For this review, take the finished solid that the model builds, in its own axes (mm). A direction names the side the tool comes from. Coordinates: 2 decimals unless noted, no trailing zeros. Order: outer loops, then holes, each group sorted by start corner. A loop starts at its lowest first (then second) coordinate and runs counter-clockwise, first axis right, second up. Notation, with made-up numbers: M 23.25,-12.75 L 50.25,-12.75 A32 ccw 50.25,17.25 Z; hole C -30,-10 d4. An arc over 180 degrees is marked long. Use CSV: the item, a comma, the result in double quotes.
```python
from build123d import *

# Parameters (mm, degrees)
ESBO_O1_R                = 5
RESSALTO_EXTRUS_O1_DEPTH = 8
ESBO_O1_3_R              = 2.5
RESSALTO_EXTRUS_O2_DEPTH = 4


with BuildPart() as part:
    # Esbo_o1 → Ressalto-extrus_o1 (new body)
    # profile 1 of 8: a face of its own
    with BuildSketch(Plane(origin=(0, 0, 0), x_dir=(1, 0, 0), z_dir=(0, 1, 0))):
        Polygon((8.06917925, -4.658742812), (8.06917925, 4.658742812), (0, 9.317485624), (-8.06917925, 4.658742812), (-8.06917925, -4.658742812), (0, -9.317485624), align=None)
        Circle(ESBO_O1_R, mode=Mode.SUBTRACT)
    # profile 2 of 8: a face of its own
    with BuildSketch(Plane(origin=(0, 0, 0), x_dir=(1, 0, 0), z_dir=(0, 1, 0))):
        Polygon((0, 9.317485624), (-4.658742812, 8.06917925), (-8.06917925, 4.658742812), align=None)
    # profile 3 of 8: a face of its own
    with BuildSketch(Plane(origin=(0, 0, 0), x_dir=(1, 0, 0), z_dir=(0, 1, 0))):
        Polygon((8.06917925, 4.658742812), (4.658742812, 8.06917925), (0, 9.317485624), align=None)
    # profile 4 of 8: a face of its own
    with BuildSketch(Plane(origin=(0, 0, 0), x_dir=(1, 0, 0), z_dir=(0, 1, 0))):
        Polygon((8.06917925, -4.658742812), (9.317485624, 0), (8.06917925, 4.658742812), align=None)
    # profile 5 of 8: a face of its own
    with BuildSketch(Plane(origin=(0, 0, 0), x_dir=(1, 0, 0), z_dir=(0, 1, 0))):
        Polygon((0, -9.317485624), (4.658742812, -8.06917925), (8.06917925, -4.658742812), align=None)
    # profile 6 of 8: a face of its own
    with BuildSketch(Plane(origin=(0, 0, 0), x_dir=(1, 0, 0), z_dir=(0, 1, 0))):
        Polygon((-8.06917925, -4.658742812), (-4.658742812, -8.06917925), (0, -9.317485624), align=None)
    # profile 7 of 8: a face of its own
    with BuildSketch(Plane(origin=(0, 0, 0), x_dir=(1, 0, 0), z_dir=(0, 1, 0))):
        Polygon((-8.06917925, 4.658742812), (-9.317485624, 0), (-8.06917925, -4.658742812), align=None)
    # profile 8 of 8: a face of its own
    with BuildSketch(Plane(origin=(0, 0, 0), x_dir=(1, 0, 0), z_dir=(0, 1, 0))):
        Circle(ESBO_O1_R)
        Polygon((4, 2.309401077), (0, 4.618802154), (-4, 2.309401077), (-4, -2.309401077), (0, -4.618802154), (4, -2.309401077), align=None, mode=Mode.SUBTRACT)
    extrude(amount=RESSALTO_EXTRUS_O1_DEPTH)

    # Esbo_o1_3 → Ressalto-extrus_o2 (add)
    with BuildSketch(Plane(origin=(0, 0, 0), x_dir=(1, 0, 0), z_dir=(0, 1, 0))):
        Polygon((4, -2.309401077), (4, 2.309401077), (0, 4.618802154), (-4, 2.309401077), (-4, -2.309401077), (0, -4.618802154), align=None)
        with Locations(Location((0, 0, 0), (0, 0, 270))):
            Circle(ESBO_O1_3_R, mode=Mode.SUBTRACT)
    extrude(amount=RESSALTO_EXTRUS_O2_DEPTH)


solid = part.part
```
Item 1: Clearance check with flat-ended pins moving along their axes: pin 1 Ø1 at (x, y) = (5.5, 4.5) entering from -Z; pin 2 Ø2.5 at (x, z) = (0, 2) entering from +Y; pin 3 Ø3 at (y, z) = (6, 6.5) entering from +X. State where each tip first meets the part, or that it passes through.
Solutions:
pin 1,"z = -7.73"
pin 2,"y = 4"
pin 3,"x = 7.73"
Item 2: Add section A-A on y = 7. State the section outline as (x, z) points.
Solutions:
outline,"M -9.32,0 L -8.07,-4.66 L -4.66,-8.07 L 0,-9.32 L 4.66,-8.07 L 8.07,-4.66 L 9.32,0 L 8.07,4.66 L 4.66,8.07 L 0,9.32 L -4.66,8.07 L -8.07,4.66 Z; hole M -4,-2.31 L 0,-4.62 L 4,-2.31 L 4,2.31 L 0,4.62 L -4,2.31 Z"
Item 3: To check wall thickness, follow line 1 along X through (y, z) = (2.9, 0); line 2 along Y through (x, z) = (-3, -2); line 3 along X through (y, z) = (2, 0.75). State the ranges of each line that lie inside material, in increasing order. Write a range as [from, to].
Solutions:
line 1,"[-9.32, -2.5], [2.5, 9.32]"
line 2,"[0, 4]"
line 3,"[-9.12, -2.38], [2.38, 9.12]"
Item 4: For faces 1 (the face through (-6.34, 3.94, -6.39)), 2 (the face through (2.028, 5.972, -3.448)), list the 3-axis set-ups (+Z, -Z, +X, -X, +Y, -Y) from which the entire face can be reached by the end or side of a thin tool; tool diameter is ignored.
Solutions:
face 1,"-Z, -X, +Y, -Y"
face 2,"+Y"
Item 5: Add section B-B on x = -0.5. State the section outline as (y, z) points, and give its area (3 significant figures).
Solutions:
outline,"M 0,-9.18 L 8,-9.18 L 8,-4.33 L 4,-4.33 L 4,-2.45 L 0,-2.45 Z; M 0,2.45 L 4,2.45 L 4,4.33 L 8,4.33 L 8,9.18 L 0,9.18 Z"
area,"92.7 mm^2"
Item 6: Add section C-C on z = 3.75. State the section outline as (x, y) points.
Solutions:
outline,"M -8.31,0 L 8.31,0 L 8.31,8 L 1.5,8 L 1.5,4 L -1.5,4 L -1.5,8 L -8.31,8 Z"
Item 7: Draft analysis for pull direction Z (two halves, no side actions). For faces 3 (the face through (2, 4, 2)), 4 (the face through (2.362, 3.944, -8.685)), 5 (the face through (8.685, 3.944, 2.362)), 6 (the face through (2, 8, 4)), state which applies: released by +Z, released by -Z, zero draft, split by the parting line, or undercut.
Solutions:
face 3,"undercut"
face 4,"released by -Z"
face 5,"released by +Z"
face 6,"zero draft"
Item 8: Add section D-D on y = 3.25. State the section outline as (x, z) points.
Solutions:
outline,"M -9.32,0 L -8.07,-4.66 L -4.66,-8.07 L 0,-9.32 L 4.66,-8.07 L 8.07,-4.66 L 9.32,0 L 8.07,4.66 L 4.66,8.07 L 0,9.32 L -4.66,8.07 L -8.07,4.66 Z; hole C 0,0 d5"
